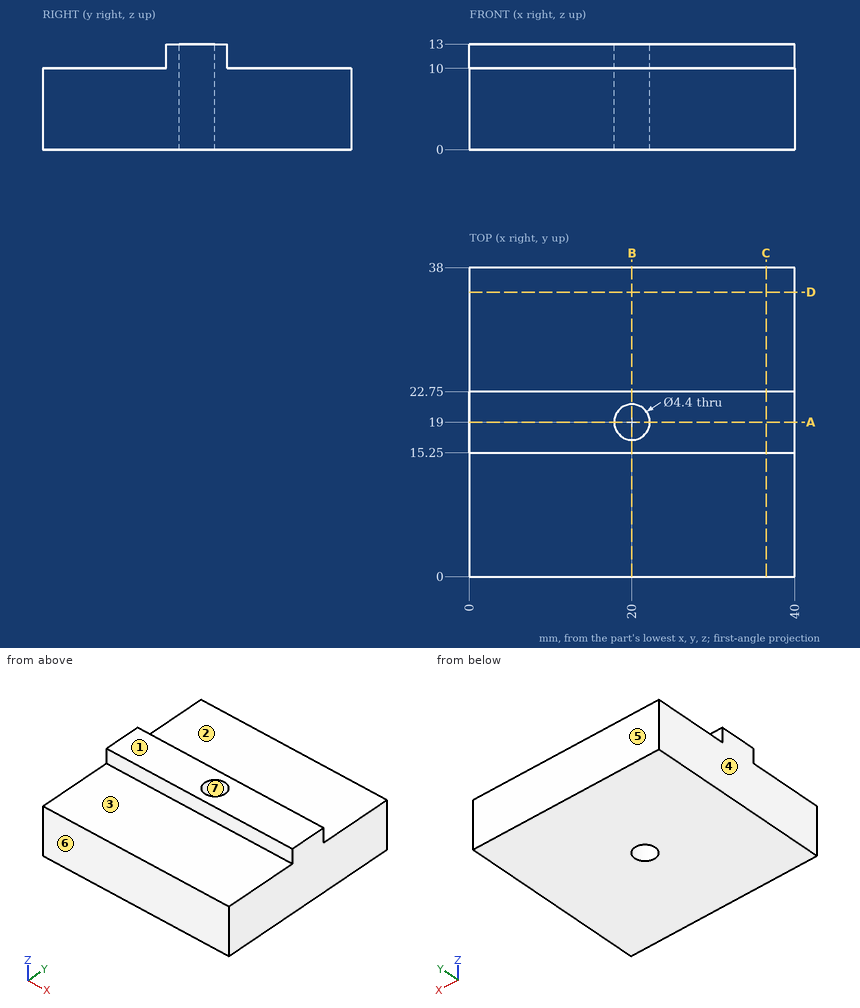
For this review, use the dimensioned drawing (mm, ordinates from the lowest corner) and the shaded views. A direction names the side the tool comes from. Give positions to 0.01 mm unless a question says otherwise; leave off trailing zeros. Write each loop counter-clockwise with the first axis right and the second up, starting at its lowest first coordinate (ties: lowest second). Pieces come first, ordered by that corner, then holes. Notation, with made-up numbers: M -32,62 L 9,62 A34 ccw 9,94 Z; hole C 10,-3 d2. An arc over 180 degrees is marked long. Answer as a JSON object with one key per item and string values. Group by question number.
Item 1: For pin 1 Ø1.5 at (x, y) = (35, 31) entering from -Z; pin 2 Ø12 at (x, y) = (13.5, 31) entering from +Z; pin 3 Ø3.5 at (x, z) = (12, 12) entering from -Y; pin 4 Ø1.5 at (x, z) = (16.5, 11.5) entering from +Y, all flat-tipped, find the tip position at first contact; note any pin that passes through.
Item 2: Tool access review of the marked faces 1, 2 and 3: name each direction out of +Z, -Z, +X, -X, +Y, -Y from which nothing blocks a thin tool from reaching the whole face with its end or side.
Item 3: Draft analysis for pull direction Y (two halves, no side actions). For the marked faces 4, 5, 6 and 7, state which applies: +Y half, -Y half, draft (parallel to the pull), parting line (faces both ways), or undercut.
Item 4: Consider section A-A on y = 19. Write out the cut boundary in (x, z), plus the area to 3 significant figures.
Item 5: Consider section D-D on y = 35. Write out the cut boundary in (x, z).
Item 6: Consider section B-B on x = 20. Write out the cut boundary in (y, z).
Item 7: For probe 1 along Y at (x, z) = (20, 7.5); probe 2 along X at (y, z) = (19, 3); probe 3 along Z at (x, y) = (35, 15), list the stretches that pass through material, from the lowest coordinate up. Write a range as [from, to].
Item 8: Consider section C-C on x = 36.5. Write out the cut boundary in (y, z).
Check result:
{
 "1": {"pin 1": "stops at z = 0", "pin 2": "stops at z = 10", "pin 3": "stops at y = 15.25", "pin 4": "stops at y = 22.75"},
 "2": {"face 1": "+Z, +X, -X, +Y, -Y", "face 2": "+Z, +X, -X, +Y", "face 3": "+Z, +X, -X, -Y"},
 "3": {"face 4": "draft", "face 5": "+Y half", "face 6": "-Y half", "face 7": "undercut"},
 "4": {"outline": "M 0,0 L 17.8,0 L 17.8,13 L 0,13 Z; M 22.2,0 L 40,0 L 40,13 L 22.2,13 Z", "area": "463 mm^2"},
 "5": {"outline": "M 0,0 L 40,0 L 40,10 L 0,10 Z"},
 "6": {"outline": "M 0,0 L 16.8,0 L 16.8,13 L 15.25,13 L 15.25,10 L 0,10 Z; M 21.2,0 L 38,0 L 38,10 L 22.75,10 L 22.75,13 L 21.2,13 Z"},
 "7": {"probe 1": "y = [0, 16.8], [21.2, 38]", "probe 2": "x = [0, 17.8], [22.2, 40]", "probe 3": "z = [0, 10]"},
 "8": {"outline": "M 0,0 L 38,0 L 38,10 L 22.75,10 L 22.75,13 L 15.25,13 L 15.25,10 L 0,10 Z"}
}
